Print and shaded views of the part. All mm, measured from the part's lowest x, y and z. Give positions to 0.01 mm unless a question says otherwise; leave off trailing zeros. Loops run counter-clockwise (first coordinate to the right, second up) from the corner with the lowest first, then second, coordinate; pieces in that order, holes last. Notation, with made-up numbers: M 58,10.25 L 104,10.25 A35 ccw 104,42.25 Z; hole C 23,74.25 d8. An arc over 180 degrees is marked long. Answer as CSV lines item,"result".
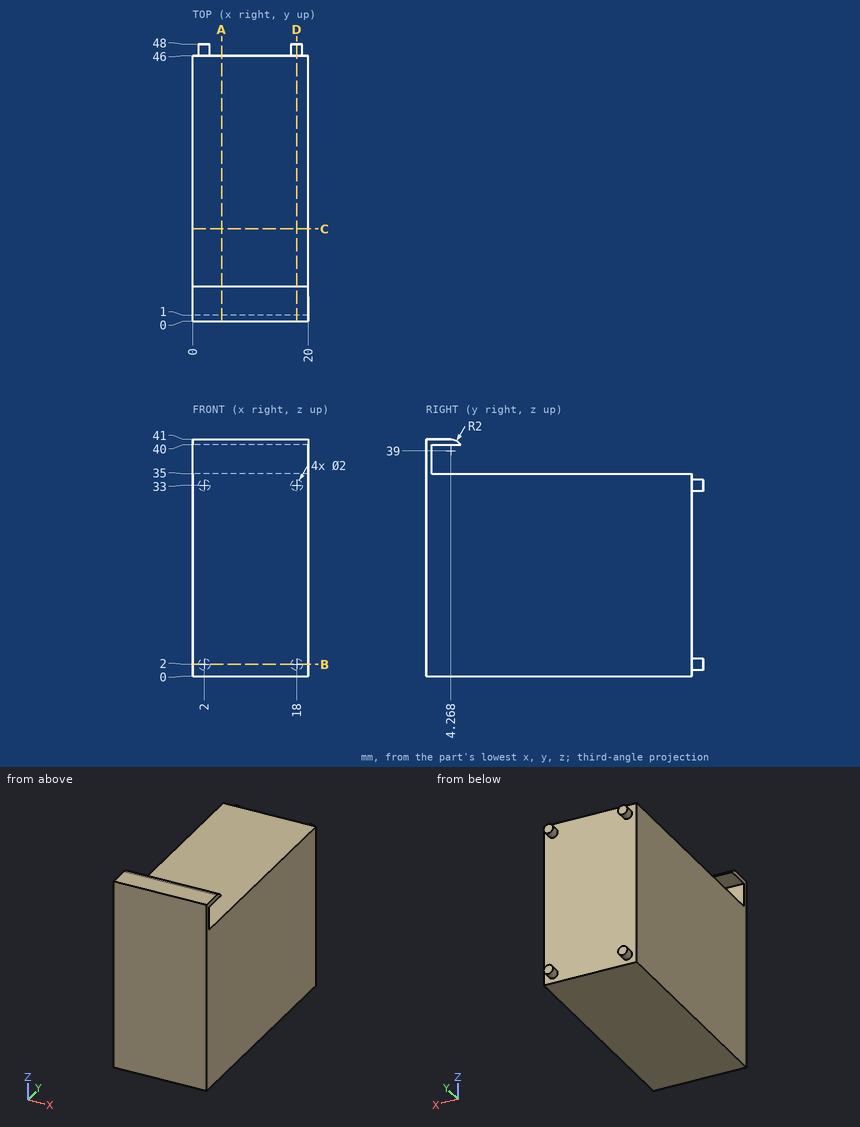
Q1. Cut at A-A (x = 5). Write the cut outline in (y, z), and give its area (3 significant figures).
Solution:
outline,"M 0,0 L 46,0 L 46,35 L 1,35 L 1,40 L 6,40 A2 ccw 4.27,41 L 0,41 Z"
area,"1,620 mm²"
Q2. Cut at D-D (x = 18). Write the cut outline in (y, z), and give its area (3 significant figures).
Solution:
outline,"M 0,0 L 46,0 L 46,1 L 48,1 L 48,3 L 46,3 L 46,32 L 48,32 L 48,34 L 46,34 L 46,35 L 1,35 L 1,40 L 6,40 A2 ccw 4.27,41 L 0,41 Z"
area,"1,630 mm²"
Q3. Cut at B-B (z = 2). Write the cut outline in (x, y).
Solution:
outline,"M 0,0 L 20,0 L 20,46 L 19,46 L 19,48 L 17,48 L 17,46 L 3,46 L 3,48 L 1,48 L 1,46 L 0,46 Z"
Q4. Wall check: line 1 (Z direction, x = 4.5, y = 10); line 2 (Y direction, x = 16, z = 14); line 3 (Y direction, x = 6.25, z = 38). Give the ranges that are in metal, low to high. Write a range as [from, to].
Solution:
line 1,"z = [0, 35]"
line 2,"y = [0, 46]"
line 3,"y = [0, 1]"
Q5. Cut at C-C (y = 16). Write the cut outline in (x, z).
Solution:
outline,"M 0,0 L 20,0 L 20,35 L 0,35 Z"
Q6. Pin check, flat tips, straight feed: P1, Ø6, axis at x = 14, y = 28, coming from the +Z side; P2, Ø1.5, axis at x = 8.5, z = 38, coming from the +Y side; P3, Ø10, axis at x = 6, z = 7, coming from the +Y side. Stop position of each tip, or through.
Solution:
P1,"stops at z = 35"
P2,"stops at y = 1"
P3,"stops at y = 46"
